from build123d import *

# Parameters (mm, degrees)
SKETCH1_W           = 20
SKETCH1_H           = 25
BOSS_EXTRUDE1_DEPTH = 20
SKETCH2_W           = 8
SKETCH2_H           = 8
CUT_EXTRUDE1_DEPTH  = 20
SKETCH3_W           = 20
SKETCH3_H           = 6
BOSS_EXTRUDE2_DEPTH = 3
LPATTERN1_COUNT     = 8
LPATTERN1_PITCH     = 23
SKETCH4_W           = 20
SKETCH4_H           = 19
BOSS_EXTRUDE3_DEPTH = 3
SKETCH5_W           = 20
SKETCH5_H           = 25
BOSS_EXTRUDE4_DEPTH = 3
SKETCH6_W           = 153
SKETCH6_H           = 2
CUT_EXTRUDE2_DEPTH  = 2
SKETCH7_W           = 187
SKETCH7_H           = 20
BOSS_EXTRUDE5_DEPTH = 7


with BuildPart() as part:
    # Sketch1 → Boss-Extrude1 (new body)
    with BuildSketch(Plane.XY):
        with Locations((10, 12.5)):
            Rectangle(SKETCH1_W, SKETCH1_H)
    extrude(amount=BOSS_EXTRUDE1_DEPTH)

    # Sketch2 → Cut-Extrude1 (cut)
    with BuildSketch(Plane.XZ):
        with Locations((10, 10)):
            Rectangle(SKETCH2_W, SKETCH2_H)
    extrude(amount=-CUT_EXTRUDE1_DEPTH, mode=Mode.SUBTRACT)

    # Sketch3 → Boss-Extrude2 (add)
    with BuildSketch(Plane(origin=(20, 0, 0), x_dir=(0, 0, -1), z_dir=(1, 0, 0))):
        with Locations((-10, 3)):
            Rectangle(SKETCH3_W, SKETCH3_H)
    extrude(amount=BOSS_EXTRUDE2_DEPTH)


with BuildPart() as lpattern1_1:
    # LPattern1: pattern copy
    add(part.part.moved(Location(Vector(1, 0, 0) * (1 * LPATTERN1_PITCH))))


with BuildPart() as lpattern1_2:
    # LPattern1: pattern copy
    add(part.part.moved(Location(Vector(1, 0, 0) * (2 * LPATTERN1_PITCH))))


with BuildPart() as lpattern1_3:
    # LPattern1: pattern copy
    add(part.part.moved(Location(Vector(1, 0, 0) * (3 * LPATTERN1_PITCH))))


with BuildPart() as lpattern1_4:
    # LPattern1: pattern copy
    add(part.part.moved(Location(Vector(1, 0, 0) * (4 * LPATTERN1_PITCH))))


with BuildPart() as lpattern1_5:
    # LPattern1: pattern copy
    add(part.part.moved(Location(Vector(1, 0, 0) * (5 * LPATTERN1_PITCH))))


with BuildPart() as lpattern1_6:
    # LPattern1: pattern copy
    add(part.part.moved(Location(Vector(1, 0, 0) * (6 * LPATTERN1_PITCH))))


with BuildPart() as lpattern1_7:
    # LPattern1: pattern copy
    add(part.part.moved(Location(Vector(1, 0, 0) * (7 * LPATTERN1_PITCH))))


with BuildPart() as lpattern1_1_1:
    add(lpattern1_1.part)

    # Combine1: union LPattern1_2, LPattern1_3, part, LPattern1_4, LPattern1_5, LPattern1_6, LPattern1_7
    add(lpattern1_2.part)
    add(lpattern1_3.part)
    add(part.part)
    add(lpattern1_4.part)
    add(lpattern1_5.part)
    add(lpattern1_6.part)
    add(lpattern1_7.part)

    # Sketch4 → Boss-Extrude3 (add)
    with BuildSketch(Plane(origin=(181, 0, 0), x_dir=(0, 0, -1), z_dir=(1, 0, 0))):
        with Locations((-10, 15.5)):
            Rectangle(SKETCH4_W, SKETCH4_H)
    extrude(amount=BOSS_EXTRUDE3_DEPTH)

    # Sketch5 → Boss-Extrude4 (add)
    with BuildSketch(Plane.ZY):
        with Locations((10, 12.5)):
            Rectangle(SKETCH5_W, SKETCH5_H)
    extrude(amount=BOSS_EXTRUDE4_DEPTH)

    # Sketch6 → Cut-Extrude2 (cut)
    with BuildSketch(Plane.XZ):
        with Locations((90.5, 10)):
            Rectangle(SKETCH6_W, SKETCH6_H)
    extrude(amount=-CUT_EXTRUDE2_DEPTH, mode=Mode.SUBTRACT)

    # Sketch7 → Boss-Extrude5 (add)
    with BuildSketch(Plane.XZ):
        with Locations((90.5, 10)):
            Rectangle(SKETCH7_W, SKETCH7_H)
    extrude(amount=BOSS_EXTRUDE5_DEPTH)


solid = lpattern1_1_1.part
Model file for the job. Use its own axes, mm. A direction names the side the tool comes from. Coordinates: 2 decimals unless noted, no trailing zeros. Order: outer loops, then holes, each group sorted by start corner. A loop starts at its lowest first (then second) coordinate and runs counter-clockwise, first axis right, second up. Notation, with made-up numbers: M -28.5,60 L -8.5,60 A22 cw -8.5,93 Z; hole C 84.25,18.25 d3. An arc over 180 degrees is marked long. Return JSON: item names as keys, results as strings.
1. Saw through at A-A (x = 80). Give the cut face in (y, z).
Ans:
{"outline": "M -7,0 L 25,0 L 25,20 L -7,20 Z; hole M 0,6 L 20,6 L 20,14 L 0,14 Z"}
2. Pull direction Z, two halves, no side cores. Call faces 3 (the face through (112, 15, 10)), 4 (the face through (102, 10, 14)): +Z half, -Z half, draft (parallel to the pull), parting line (faces both ways), or undercut.
Ans:
{"face 3": "draft", "face 4": "undercut"}
3. Flat gauge pin, fed straight in: pin 1 (1 mm diameter, centred on x = 117, y = 1, fed in from -Z). Where does the tip first touch, or does it go through?
Ans:
{"pin 1": "z = 0"}
4. Drill centre lines: probe 1 along Y at (x, z) = (139.5, 10.25); probe 2 along Y at (x, z) = (78, 13); probe 3 along Z at (x, y) = (168, 14.5). Where is each one in solid material? Low to high.
Ans:
{"probe 1": "-7 to 0, 2 to 25", "probe 2": "-7 to 0, 20 to 25", "probe 3": "0 to 6, 14 to 20"}
5. Tool access for faces 1 (the face through (144, 10, 10)), 2 (the face through (69, 15, 10)): list every direction of +Z, -Z, +X, -X, +Y, -Y with a clear straight run to the whole face (end or side of a thin tool).
Ans:
{"face 1": "none", "face 2": "+Z, -Z, +Y"}
6. Saw through at B-B (y = 10.5). Give the number of separate pieces and of enclosed holes in the cut face, and give its area (3 significant figures).
Ans:
{"separate pieces": "8", "enclosed holes": "8", "area": "2,810 mm^2"}
